For this review, take the finished solid that the model builds, in its own axes (mm). Give positions to 0.01 mm unless a question says otherwise; leave off trailing zeros. Loops run counter-clockwise (first coordinate to the right, second up) from the corner with the lowest first, then second, coordinate; pieces in that order, holes last. Notation, with made-up numbers: (-13, 15.5) - (36, 15.5) arc R30 ccw to (36, 44.5) - close; hole circle Ø10 at (57, -3.75). An arc over 180 degrees is marked (long way). Answer in a Markdown table with one row per item.
```python
from build123d import *

# Parameters (mm, degrees)
SKETCH_1_R          = 22.5
SKETCH_1_R_2        = 12.5
EXTRUDE_1_DEPTH     = 2
SKETCH_2_R          = 1.25
CUT_EXTRUDE_1_DEPTH = 2


with BuildPart() as part:
    # Эскиз1 → Бобышка-Вытянуть1 (new body)
    with BuildSketch(Plane(origin=(0, 0, 0), x_dir=(1, 0, 0), z_dir=(0, 1, 0))):
        with Locations(Location((0, 0, 0), (0, 0, 270))):
            Circle(SKETCH_1_R)
        with Locations(Location((0, 0, 0), (0, 0, 270))):
            Circle(SKETCH_1_R_2, mode=Mode.SUBTRACT)
    extrude(amount=EXTRUDE_1_DEPTH)

    # Эскиз2 → Вырез-Вытянуть1 (cut)
    with BuildSketch(Plane(origin=(0, 2, 0), x_dir=(1, 0, 0), z_dir=(0, 1, 0))):
        with Locations(Location((-19, 0, 0), (0, 0, 270))):
            Circle(SKETCH_2_R)
        with Locations(Location((19, 0, 0), (0, 0, 270))):
            Circle(SKETCH_2_R)
        with Locations(Location((0, -19, 0), (0, 0, 270))):
            Circle(SKETCH_2_R)
        Polygon((-20.23493598, 18), (18.121302114, 18), (0, 26.542268098), align=None)
    extrude(amount=-CUT_EXTRUDE_1_DEPTH, mode=Mode.SUBTRACT)


solid = part.part
```
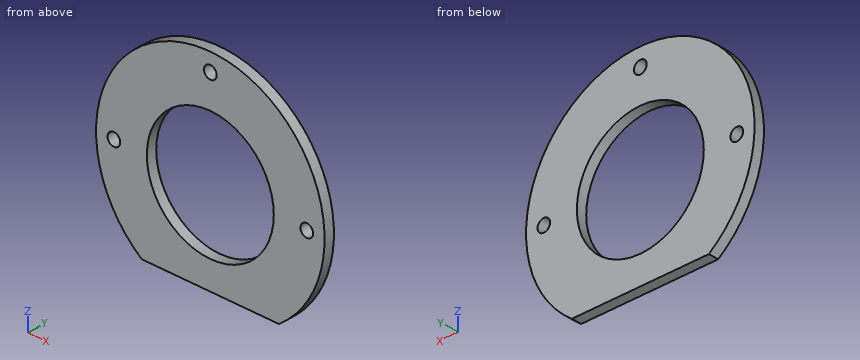
1. We need section D-D, the plane x = -6. Give the boundary of the cut face in (y, z), and give its area (3 significant figures).
Values:
| item | result |
|---|---|
| outline | (0, -18) - (2, -18) - (2, -10.97) - (0, -10.97) - close; (0, 10.97) - (2, 10.97) - (2, 21.69) - (0, 21.69) - close |
| area | 35.5 mm^2 |
2. We need section C-C, the plane y = 1.1. Give the boundary of the cut face in (x, z), and give its area (3 significant figures).
Values:
| item | result |
|---|---|
| outline | (-13.5, -18) - (13.5, -18) arc R22.5 ccw (long way) to start; hole circle Ø2.5 at (-19, 0); hole circle Ø25 at (0, 0); hole circle Ø2.5 at (0, 19); hole circle Ø2.5 at (19, 0) |
| area | 1,000 mm^2 |
3. We need section B-B, the plane z = -8. Give the boundary of the cut face in (x, y), and give its area (3 significant figures).
Values:
| item | result |
|---|---|
| outline | (-21.03, 0) - (-9.6, 0) - (-9.6, 2) - (-21.03, 2) - close; (9.6, 0) - (21.03, 0) - (21.03, 2) - (9.6, 2) - close |
| area | 45.7 mm^2 |
4. Clearance check with flat-ended pins moving along their axes: pin 1 (2 mm diameter, centred on x = 0, z = 19, fed in from -Y); pin 2 (1 mm diameter, centred on y = 0.5, z = 2.5, fed in from -X). State where each tip first meets the part, or that it passes through.
Values:
| item | result |
|---|---|
| pin 1 | passes through |
| pin 2 | stops at x = -22.41 |
5. We need section A-A, the plane x = 0. Give the boundary of the cut face in (y, z), and give its area (3 significant figures).
Values:
| item | result |
|---|---|
| outline | (0, -18) - (2, -18) - (2, -12.5) - (0, -12.5) - close; (0, 12.5) - (2, 12.5) - (2, 17.75) - (0, 17.75) - close; (0, 20.25) - (2, 20.25) - (2, 22.5) - (0, 22.5) - close |
| area | 26.0 mm^2 |
6. Wall thickness on line 1 (X direction, y = 1.45, z = 0); line 2 (Z direction, x = -1, y = 0.35); line 3 (X direction, y = 1.2, z = 19): over which ranges is each line inside the solid? List them lowest first. Write a range as [from, to].
Values:
| item | result |
|---|---|
| line 1 | x = [-22.5, -20.25], [-17.75, -12.5], [12.5, 17.75], [20.25, 22.5] |
| line 2 | z = [-18, -12.46], [12.46, 18.25], [19.75, 22.48] |
| line 3 | x = [-12.05, -1.25], [1.25, 12.05] |
